from build123d import *

# Parameters (mm, degrees)
BOSS_EXTRUDE1_DEPTH = 21.2
SKETCH2_R           = 12.5
BOSS_EXTRUDE2_DEPTH = 7.5
SKETCH3_R           = 3
CUT_EXTRUDE1_DEPTH  = 5


with BuildPart() as part:
    # Sketch1 → Boss-Extrude1 (new body)
    with BuildSketch(Plane.XY):
        with BuildLine():
            Line((-28.25, -21), (28.25, -21))
            ThreePointArc((28.25, -21), (29.664213562, -20.414213562), (30.25, -19))
            Line((30.25, -19), (30.25, 19))
            ThreePointArc((30.25, 19), (29.664213562, 20.414213562), (28.25, 21))
            Line((28.25, 21), (-28.25, 21))
            ThreePointArc((-28.25, 21), (-29.664213562, 20.414213562), (-30.25, 19))
            Line((-30.25, 19), (-30.25, -19))
            ThreePointArc((-30.25, -19), (-29.664213562, -20.414213562), (-28.25, -21))
        make_face()
    extrude(amount=BOSS_EXTRUDE1_DEPTH)

    # Sketch2 → Boss-Extrude2 (add)
    with BuildSketch(Plane.XY.offset(21.2)):
        with Locations((13.25, 0)):
            Circle(SKETCH2_R)
    extrude(amount=BOSS_EXTRUDE2_DEPTH)

    # Sketch3 → Cut-Extrude1 (cut)
    with BuildSketch(Plane.XZ.offset(21)):
        with Locations(Location((13.25, 10, 0), (0, 0, 270))):
            Circle(SKETCH3_R)
    extrude(amount=-CUT_EXTRUDE1_DEPTH, mode=Mode.SUBTRACT)


solid = part.part
For this review, take the finished solid that the model builds, in its own axes (mm). A direction names the side the tool comes from. Give positions to 0.01 mm unless a question says otherwise; leave off trailing zeros. Order: outer loops, then holes, each group sorted by start corner. A loop starts at its lowest first (then second) coordinate and runs counter-clockwise, first axis right, second up. Notation, with made-up numbers: M 72.25,80 L 105.25,80 A36 ccw 105.25,118 Z; hole C 33.5,-32 d2. An arc over 180 degrees is marked long. Answer in a Markdown table with one row per item. Add a question column.
(1) Consider section D-D on y = 8.5. State the section outline as (x, z) points.
(2) Mouldability with a two-part tool opening along X and no side actions: class faces 1 (the face through (13, 0, 28.7)), 2 (the face through (-29.65, 20.43, 10.45)), 3 (the face through (10.32, -18.54, 10.65)) as +X half, -X half, draft (parallel to the pull), parting line (faces both ways), or undercut.
(3) Consider section C-C on z = 23.75. State the section outline as (x, y) points.
(4) Wall thickness on probe 1 along X at (y, z) = (-18.9, 10); probe 2 along Z at (x, y) = (13, -17); probe 3 along Z at (x, y) = (-21, 11): over which ranges is each line inside the solid? List them lowest first. Write a range as [from, to].
(5) Consider section B-B on x = 13.25. State the section outline as (y, z) points.
(6) Consider section A-A on y = 0. State the section outline as (x, z) points, and give its area (3 significant figures).
(7) For faces 4 (the face through (29.65, -20.43, 10.45)), 5 (the face through (0.762, 0.55, 24.898)), 6 (the face through (13, -16, 10)), list the 3-axis set-ups (+Z, -Z, +X, -X, +Y, -Y) from which the entire face can be reached by the end or side of a thin tool; tool diameter is ignored.
(8) For pin 1 (1.8 mm diameter, centred on x = 14, z = 11, fed in from -Y); pin 2 (2 mm diameter, centred on x = 24, y = 13, fed in from +Z); pin 3 (1 mm diameter, centred on x = -20, z = 23, fed in from +Y), all flat-tipped, find the tip position at first contact; note any pin that passes through.
Evaluation:
| question | item | result |
|---|---|---|
| 1 | outline | M -30.25,0 L 30.25,0 L 30.25,21.2 L 22.42,21.2 L 22.42,28.7 L 4.08,28.7 L 4.08,21.2 L -30.25,21.2 Z |
| 2 | face 1 | draft |
| 2 | face 2 | -X half |
| 2 | face 3 | undercut |
| 3 | outline | C 13.25,0 d25 |
| 4 | probe 1 | x = [-30.25, 10.25], [16.25, 30.25] |
| 4 | probe 2 | z = [0, 7.01], [12.99, 21.2] |
| 4 | probe 3 | z = [0, 21.2] |
| 5 | outline | M -21,0 L 21,0 L 21,21.2 L 12.5,21.2 L 12.5,28.7 L -12.5,28.7 L -12.5,21.2 L -21,21.2 L -21,13 L -16,13 L -16,7 L -21,7 Z |
| 6 | outline | M -30.25,0 L 30.25,0 L 30.25,21.2 L 25.75,21.2 L 25.75,28.7 L 0.75,28.7 L 0.75,21.2 L -30.25,21.2 Z |
| 6 | area | 1,470 mm^2 |
| 7 | face 4 | +Z, -Z, +X, -Y |
| 7 | face 5 | +Z |
| 7 | face 6 | -Y |
| 8 | pin 1 | stops at y = -16 |
| 8 | pin 2 | stops at z = 21.2 |
| 8 | pin 3 | passes through |
